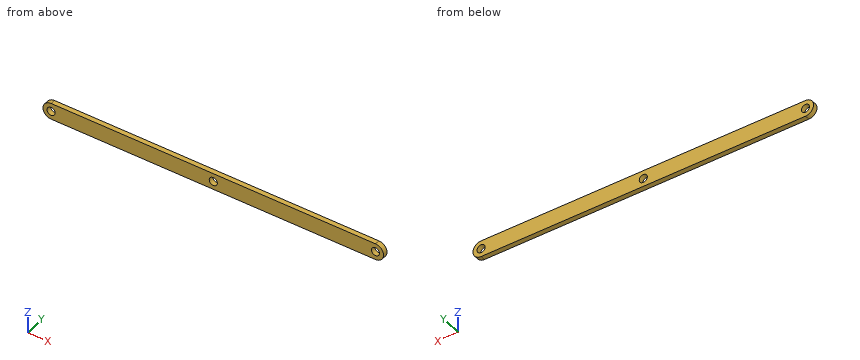
from build123d import *

# Parameters (mm, degrees)
BOSS_EXTRUDE1_DEPTH = 3
CUT_EXTRUDE1_REACH  = 107.162
SKETCH3_R           = 2.5
CUT_EXTRUDE2_REACH  = 107.162
SKETCH5_R           = 2.5


with BuildPart() as part:
    # Sketch2 → Boss-Extrude1 (new body)
    with BuildSketch(Plane(origin=(0, 0, 0), x_dir=(1, 0, 0), z_dir=(0, 1, 0))):
        with BuildLine():
            Line((-100, 5), (100, 5))
            ThreePointArc((100, 5), (105, 0), (100, -5))
            Line((100, -5), (-100, -5))
            ThreePointArc((-100, -5), (-105, 0), (-100, 5))
        make_face()
    extrude(amount=BOSS_EXTRUDE1_DEPTH)

    # Sketch3 → Cut-Extrude1 (cut, up to next)
    with BuildSketch(Plane(origin=(0, 3, 0), x_dir=(1, 0, 0), z_dir=(0, 1, 0)), mode=Mode.PRIVATE) as cut_extrude1_sk1:
        with Locations(Location((100, 0, 0), (0, 0, 270))):
            Circle(SKETCH3_R)
    cut_extrude1_tool1 = extrude(cut_extrude1_sk1.sketch, amount=-CUT_EXTRUDE1_REACH, mode=Mode.PRIVATE) & part.part
    cut_extrude1 = cut_extrude1_tool1.solids().sort_by_distance((100, 3, 0))[0]
    add(cut_extrude1, mode=Mode.SUBTRACT)

    # Mirror1: Cut-Extrude1 across plane
    add(cut_extrude1.mirror(Plane(origin=(0, 0, 0), x_dir=(0, 0, 1), z_dir=(1, 0, 0))), mode=Mode.SUBTRACT)

    # Sketch5 → Cut-Extrude2 (cut, up to next)
    with BuildSketch(Plane.XZ, mode=Mode.PRIVATE) as cut_extrude2_sk1:
        with Locations(Location((0, 0, 0), (0, 0, 270))):
            Circle(SKETCH5_R)
    cut_extrude2_tool1 = extrude(cut_extrude2_sk1.sketch, amount=-CUT_EXTRUDE2_REACH, mode=Mode.PRIVATE) & part.part
    add(cut_extrude2_tool1.solids().sort_by_distance((0, 0, 0))[0], mode=Mode.SUBTRACT)


solid = part.part
Here's how the part is built. I have some questions about the finished solid (model axes, mm). Round coordinates to 2 decimals unless told otherwise and drop trailing zeros. Loops run counter-clockwise (first coordinate to the right, second up) from the corner with the lowest first, then second, coordinate; pieces in that order, holes last. Notation, with made-up numbers: (29.25, 78.25) - (74.25, 78.25) arc R18 cw to (74.25, 100.25) - close; hole circle Ø10 at (29.5, -36.75). An arc over 180 degrees is marked (long way). One line per question, with ' | ' between items. Start each with the question number.
Q1. I want a section at C-C (y = 0.9). Write out the boundary of the cut face in (x, z), then the cut area to 3 significant figures.
Q2. I want a section at A-A (z = 0). Write out the boundary of the cut face in (x, y).
Q3. Will this pin go through, and if not, where does the flat tip stop? pin 1 (4.5 mm diameter, centred on x = 0, z = 0, fed in from +Y).
Q4. Please list where these lines run through material, in increasing order: line 1 (X direction, y = 0.8, z = -0.25); line 2 (Z direction, x = -100, y = 0.9); line 3 (X direction, y = 1.25, z = 4). Write a range as [from, to].
Q5. I want a section at B-B (x = 0). Write out the boundary of the cut face in (y, z).
Response values:
1) outline: (-100, -5) - (100, -5) arc R5 ccw to (100, 5) - (-100, 5) arc R5 ccw to start; hole circle Ø5 at (-100, 0); hole circle Ø5 at (0, 0); hole circle Ø5 at (100, 0) | area: 2,020 mm²
2) outline: (-105, 0) - (-102.5, 0) - (-102.5, 3) - (-105, 3) - close; (-97.5, 0) - (-2.5, 0) - (-2.5, 3) - (-97.5, 3) - close; (2.5, 0) - (97.5, 0) - (97.5, 3) - (2.5, 3) - close; (102.5, 0) - (105, 0) - (105, 3) - (102.5, 3) - close
3) pin 1: passes through
4) line 1: x = [-104.99, -102.49], [-97.51, -2.49], [2.49, 97.51], [102.49, 104.99] | line 2: z = [-5, -2.5], [2.5, 5] | line 3: x = [-103, 103]
5) outline: (0, -5) - (3, -5) - (3, -2.5) - (0, -2.5) - close; (0, 2.5) - (3, 2.5) - (3, 5) - (0, 5) - close
